Autodesk Fusion 360 part; units mm, degrees
sketch "Sketch2" plane through (0, 0, 0) normal (0, 1, 0) x (1, 0, 0)
  line L0 (0, 0) -> (-28, 0)
  line L1 (-28, 0) -> (-28, 28)
  line L2 (-28, 28) -> (0, 28)
  line L3 (0, 28) -> (0, 0)
  dimension "d1" = 28
  dimension "d2" = 28
extrude "Extrude1" add sketch "Sketch2" along normal blind 1435
sketch "Sketch3" plane through (0, 0, -28) normal (0, 0, -1) x (-1, 0, 0)
  line L0 (0, 0) -> (28, 0)
  line L1 (28, 0) -> (28, 1435)
  line L2 (28, 1435) -> (0, 1435)
  line L3 (0, 1435) -> (0, 0)
  circle A0 centre (13, 1420) radius 6
  line L4 (28, 717.5) -> (0, 717.5) construction
  circle A1 centre (13, 15) radius 6
  dimension "d5" = 12
  dimension "d6" = 15
  dimension "d7" = 15
extrude "Extrude2" cut sketch "Sketch3" against normal through all contours A0 | A1
fillet "Fillet1" radius 0.5 12 edges at (-28, 717.5, 0) (0, 717.5, 0) (-28, 717.5, -28) (0, 717.5, -28) (0, 1435, -14) (-14, 1435, -28) (-28, 1435, -14) (-14, 1435, 0) (-14, 0, 0) (-28, 0, -14) (0, 0, -14) (-14, 0, -28)
equation "d7 = d6"
Source: CAD feature listing. Evaluate the final solid. Frame: model axes, mm. Round coordinates to 2 decimals unless told otherwise and drop trailing zeros. Write each loop counter-clockwise with the first axis right and the second up, starting at its lowest first coordinate (ties: lowest second). Pieces come first, ordered by that corner, then holes. Notation, with made-up numbers: M -33.5,5.5 L -20.5,5.5 A19 cw -20.5,27.5 Z; hole C 43.25,35.25 d6. An arc over 180 degrees is marked long. Answer as a JSON object with one key per item and string values. Group by question number.
(1) Section query A-A on x = -13. Output: boundary loops of the cut face in (y, z), then the cut area to 3 significant figures.
(2) Ray query, line 1 (Y direction, x = -13, z = -14); line 2 (Y direction, x = -11.5, z = -9.5); line 3 (X direction, y = 1420, z = -19.5). Return the intervals inside material, ascending. Write a range as [from, to].
(3) Mould query, pull axis Y, two halves, no side actions, for faces 1 (the flat face through (-14, 1435, -14)), 2 (the flat face through (-14, 707, 0)), 3 (the flat face through (-14, 0, -14)). Classes: +Y half, -Y half, draft (parallel to the pull), parting line (faces both ways), or undercut.
Computed values:
{
 "1": {"outline": "M 0,-27.5 A0.5 ccw 0.5,-28 L 9,-28 L 9,0 L 0.5,0 A0.5 ccw 0,-0.5 Z; M 21,-28 L 1414,-28 L 1414,0 L 21,0 Z; M 1426,-28 L 1434.5,-28 A0.5 ccw 1435,-27.5 L 1435,-0.5 A0.5 ccw 1434.5,0 L 1426,0 Z", "area": "39,500 mm^2"},
 "2": {"line 1": "[0, 9], [21, 1414], [1426, 1435]", "line 2": "[0, 9.19], [20.81, 1414.19], [1425.81, 1435]", "line 3": "[-28, -19], [-7, 0]"},
 "3": {"face 1": "+Y half", "face 2": "draft", "face 3": "-Y half"}
}
